Work out the finished part from the listing and answer in its coordinate system (mm). Round coordinates to 2 decimals unless told otherwise and drop trailing zeros. Order: outer loops, then holes, each group sorted by start corner. A loop starts at its lowest first (then second) coordinate and runs counter-clockwise, first axis right, second up. Notation, with made-up numbers: (60, 76.25) - (99, 76.25) arc R13 cw to (99, 90.25) - close; hole circle Ø7 at (-14.5, -27.75). An arc over 180 degrees is marked (long way). Answer in a Markdown table with one row per item.
Autodesk Inventor part; units mm, degrees
ref_plane "YZ Plane" through (0, 0, 0) normal (1, 0, 0) x (0, 1, 0)
ref_plane "XZ Plane" through (0, 0, 0) normal (0, 1, 0) x (-1, 0, 0)
ref_plane "XY Plane" through (0, 0, 0) normal (0, 0, 1) x (1, 0, 0)
sketch "Sketch1" plane through (0, 0, 0) normal (0, 0, 1) x (1, 0, 0)
  line L0 (-1498, 0) -> (1498, 0) construction
  line L1 (-1498, 0) -> (-898, 0)
  line L2 (-898, 0) -> (-898, 2068)
  line L3 (-898, 2068) -> (-1498, 2068)
  line L4 (-1498, 2068) -> (-1498, 0)
  line L5 (-898, 0) -> (-498, 0)
  line L6 (-498, 0) -> (-498, 816)
  line L7 (-498, 816) -> (-898, 816)
  line L8 (-898, 816) -> (-898, 0)
  line L9 (-498, 0) -> (102, 0)
  line L10 (102, 0) -> (102, 816)
  line L11 (102, 816) -> (-498, 816)
  line L12 (-498, 816) -> (-498, 0)
  line L13 (102, 0) -> (698, 0)
  line L14 (698, 0) -> (698, 668)
  line L15 (698, 668) -> (102, 668)
  line L16 (102, 668) -> (102, 0)
  line L17 (698, 0) -> (1498, 0)
  line L18 (1498, 0) -> (1498, 816)
  line L19 (1498, 816) -> (698, 816)
  line L20 (698, 816) -> (698, 0)
  line L21 (-1498, 0) -> (1498, 0)
  line L22 (1498, 0) -> (1498, 96)
  line L23 (1498, 96) -> (-1498, 96)
  line L24 (-1498, 96) -> (-1498, 0)
  line L25 (-898, 816) -> (1498, 816)
  line L26 (1498, 816) -> (1498, 832)
  line L27 (1498, 832) -> (-898, 832)
  line L28 (-898, 832) -> (-898, 816)
  line L29 (-898, 1972) -> (-498, 1972)
  line L30 (-498, 1972) -> (-498, 1372)
  line L31 (-498, 1372) -> (-898, 1372)
  line L32 (-898, 1372) -> (-898, 1972)
  line L33 (698, 1972) -> (1498, 1972)
  line L34 (1498, 1972) -> (1498, 1372)
  line L35 (1498, 1372) -> (698, 1372)
  line L36 (698, 1372) -> (698, 1972)
  line L37 (698, 1372) -> (98, 1372)
  line L38 (98, 1372) -> (98, 1972)
  line L39 (98, 1972) -> (698, 1972)
  line L40 (698, 1972) -> (698, 1372)
  line L41 (-498, 1372) -> (98, 1372)
  line L42 (-498, 1372) -> (-275, 1637.7611)
  line L43 (98, 1372) -> (-125, 1637.7611)
  line L44 (-275, 1637.7611) -> (-125, 1637.7611)
  line L45 (-125, 1637.7611) -> (-125, 2068)
  line L46 (-125, 2068) -> (-275, 2068)
  line L47 (-275, 2068) -> (-275, 1637.7611)
  line L48 (1098, 816) -> (1098, 96)
  line L49 (-198, 816) -> (-198, 96)
  line L50 (-898, 668) -> (-498, 668)
  line L51 (-1498, 520) -> (-898, 520)
  line L52 (-1498, 1579) -> (-898, 1579)
  line L53 (398, 1972) -> (398, 1372)
  line L54 (1098, 1972) -> (1098, 1372)
  line L55 (698, 1876) -> (1498, 1876)
  line L56 (698, 1468) -> (1498, 1468)
  line L57 (-1498, 1049.5) -> (-898, 1049.5)
  line L58 (1498, 832) -> (1514, 832)
  line L59 (1514, 832) -> (1514, 816)
  line L60 (1514, 816) -> (1498, 816)
  line L61 (1498, 816) -> (1498, 832)
  point P0 (0, 0)
  point P1 (0, 0)
  point P2 (0, 0)
  point P3 (-198, 816)
  point P4 (0, 0)
  dimension "d0" = 2996
  dimension "d1" = 600
  dimension "d2" = 2068
  dimension "d3" = 400
  dimension "d4" = 816
  dimension "d5" = 600
  dimension "d6" = 816
  dimension "d7" = 596
  dimension "d8" = 668
  dimension "d9" = 800
  dimension "d10" = 816
  dimension "d11" = 96
  dimension "d12" = 16
  dimension "d13" = 400
  dimension "d14" = 600
  dimension "d15" = 96
  dimension "d16" = 800
  dimension "d17" = 600
  dimension "d18" = 600
  dimension "d19" = 600
  dimension "d20" = 50
  dimension "d21" = 150
  dimension "d22" = 148
  dimension "d23" = 1059
  dimension "d24" = 96
  dimension "d25" = 96
  dimension "d26" = 529.5
  dimension "d27" = 16
extrude "Extrusion1" add sketch "Sketch1" along normal blind 476 contours L2 L27 L26 L19 L25 L11 L7 | L58 L59 L60 L26
fillet "Fillet1" radius 4 4 edges at (300, 832, 476) (-698, 816, 476) (1514, 832, 238) (1514, 816, 238)
sketch "Sketch2" plane through (-898, 832, 0) normal (0, 1, 0) x (1, 0, 0)
  line L0 (2408, -472) -> (0, -472)
  line L1 (400, 0) -> (1000, 0)
  line L2 (1000, 0) -> (1000, -472)
  line L3 (1000, -472) -> (400, -472)
  line L4 (400, -472) -> (400, 0)
  line L5 (1596, 0) -> (2396, 0)
  line L6 (2396, 0) -> (2396, -472)
  line L7 (2396, -472) -> (1596, -472)
  line L8 (1596, -472) -> (1596, 0)
  line L9 (950, -422) -> (950, -50)
  line L10 (950, -50) -> (450, -50)
  line L11 (450, -50) -> (450, -422)
  line L12 (450, -422) -> (950, -422)
  line L13 (2346, -50) -> (1646, -50)
  line L14 (1646, -50) -> (1646, -422)
  line L15 (1646, -422) -> (2346, -422)
  line L16 (2346, -422) -> (2346, -50)
  point P0 (898, 0)
  point P1 (400, 0)
  point P2 (1000, 0)
  point P3 (1596, 0)
  point P4 (2396, 0)
  dimension "d31" = 50
  dimension "d32" = 50
extrude "Extrusion2" cut sketch "Sketch2" against normal blind 20 contours L12 L11 L10 L9 | L16 L15 L14 L13
properties part number "Countertop"
1) Find the intervals of material crossed by probe 1 along X at (y, z) = (821.25, 139); probe 2 along X at (y, z) = (829.25, 157); probe 3 along Z at (x, y) = (-431.5, 822.5), in increasing order. Write a range as from..to.
Filled in:
| item | result |
|---|---|
| probe 1 | x = -898..-448, 52..748, 1448..1514 |
| probe 2 | x = -898..-448, 52..748, 1448..1513.8 |
| probe 3 | z = 0..50, 422..476 |
2) Each of these flat-tipped pins is pushed along its axis until it touches: pin 1 (4 mm diameter, centred on x = 212.5, y = 830, fed in from +Z); pin 2 (3 mm diameter, centred on y = 830, z = 145, fed in from +X). Where does it stop, or does it pass through?
Filled in:
| item | result |
|---|---|
| pin 1 | stops at z = 476 |
| pin 2 | stops at x = 1513.97 |
3) Find section C-C, the plane y = 823.25. Give the vertices of the cut face in (x, z), then the cut area to 3 significant figures.
Filled in:
| item | result |
|---|---|
| outline | (-898, 0) - (1514, 0) - (1514, 476) - (-898, 476) - close; hole (-448, 50) - (52, 50) - (52, 422) - (-448, 422) - close; hole (748, 50) - (1448, 50) - (1448, 422) - (748, 422) - close |
| area | 702,000 mm^2 |
4) Find section B-B, the plane z = 100. Give the vertices of the cut face in (x, y), then the cut area to 3 significant figures.
Filled in:
| item | result |
|---|---|
| outline | (-898, 816) - (-448, 816) - (-448, 832) - (-898, 832) - close; (52, 816) - (748, 816) - (748, 832) - (52, 832) - close; (1448, 816) - (1510, 816) arc R4 ccw to (1514, 820) - (1514, 828) arc R4 ccw to (1510, 832) - (1448, 832) - close |
| area | 19,400 mm^2 |
5) Find section A-A, the plane x = 932.5. Give the vertices of the cut face in (y, z), then the cut area to 3 significant figures.
Filled in:
| item | result |
|---|---|
| outline | (816, 0) - (832, 0) - (832, 50) - (816, 50) - close; (816, 422) - (832, 422) - (832, 472) arc R4 ccw to (828, 476) - (820, 476) arc R4 ccw to (816, 472) - close |
| area | 1,660 mm^2 |
